Build history of the part. All positions in model axes, mm. A direction names the side the tool comes from. Coordinates: 2 decimals unless noted, no trailing zeros. Loops run counter-clockwise (first coordinate to the right, second up) from the corner with the lowest first, then second, coordinate; pieces in that order, holes last.
Item 1: Cut at A-A (y = 0). List the corners of the cut face in (x, z), and give its area (3 significant figures).
Item 2: Cut at C-C (x = 73.5). List the corners of the cut face in (y, z), and give its area (3 significant figures).
Item 3: Flat gauge pins, fed straight in: pin 1 (12 mm diameter, centred on y = -3.5, z = 58.5, fed in from +X); pin 2 (6.5 mm diameter, centred on x = 44.5, y = 28.5, fed in from -Z); pin 3 (5 mm diameter, centred on x = 4.5, z = 0, fed in from -Y). Where does each tip first touch, or does it go through?
Item 4: 3-axis set-ups, long thin cutter, end or side, ignore diameter. For faces 4 (the face through (5, -20, 1)), 5 (the face through (86, 11.6, 22.5)), 6 (the face through (49, 32.495, 0)): which of +Z, -Z, +X, -X, +Y, -Y reach the whole face in a straight line?
Item 5: Mould opens along Z. For faces 1 (the face through (17.75, -28.73, -69.28)), 2 (the face through (49, 28, 5)), 3 (the face through (10, 0, -45)) say: released by +Z, released by -Z, zero draft, split by the parting line, or undercut.
Item 6: Drill centre lines: line 1 along Y through (x, z) = (70, 0); line 2 along Y through (x, z) = (35.5, 0); line 3 along Z through (x, y) = (26, 0). Where is each one in solid material? Low to high.
Item 7: Cut at D-D (x = 23.5). List the corners of the cut face in (y, z), and give its area (3 significant figures).
Item 8: Cut at B-B (z = 0). List the corners of the cut face in (x, y), and give its area (3 significant figures).
from build123d import *

# Parameters (mm, degrees)
SKETCH1_R           = 75
BOSS_EXTRUDE1_DEPTH = 36
SKETCH2_R           = 50
BOSS_EXTRUDE2_DEPTH = 50
CUT_EXTRUDE2_DEPTH  = 10
CUT_EXTRUDE3_DEPTH  = 76
CHAMFER1_SIZE       = 1
CHAMFER2_SIZE       = 1


with BuildPart() as part:
    # Sketch1 → Boss-Extrude1 (new body)
    with BuildSketch(Plane(origin=(0, 0, 0), x_dir=(0, 0, -1), z_dir=(1, 0, 0))):
        Circle(SKETCH1_R)
    extrude(amount=BOSS_EXTRUDE1_DEPTH)

    # Sketch2 → Boss-Extrude2 (add)
    with BuildSketch(Plane(origin=(36, 0, 0), x_dir=(0, 0, -1), z_dir=(1, 0, 0))):
        Circle(SKETCH2_R)
    extrude(amount=BOSS_EXTRUDE2_DEPTH)

    # Sketch4 → Cut-Extrude2 (cut)
    with BuildSketch(Plane.ZY):
        with BuildLine():
            Line((-72.284161474, 20), (72.284161474, 20))
            ThreePointArc((72.284161474, 20), (75, 0), (72.284161474, -20))
            Line((72.284161474, -20), (-72.284161474, -20))
            ThreePointArc((-72.284161474, -20), (-75, 0), (-72.284161474, 20))
        make_face()
    extrude(amount=-CUT_EXTRUDE2_DEPTH, mode=Mode.SUBTRACT)

    # Sketch5 → Cut-Extrude3 (cut)
    with BuildSketch(Plane(origin=(86, 0, 0), x_dir=(0, 0, -1), z_dir=(1, 0, 0))):
        with BuildLine():
            Line((-5, 32.494897428), (5, 32.494897428))
            Line((5, 32.494897428), (5, 24.494897428))
            ThreePointArc((5, 24.494897428), (0, -25), (-5, 24.494897428))
            Line((-5, 24.494897428), (-5, 32.494897428))
        make_face()
    extrude(amount=-CUT_EXTRUDE3_DEPTH, mode=Mode.SUBTRACT)

    # Chamfer1
    chamfer1_edges = [part.edges().sort_by_distance(p)[0] for p in [
        (86, 0, 50),
    ]]
    chamfer(chamfer1_edges, length=CHAMFER1_SIZE)

    # Chamfer2
    chamfer2_edges = [part.edges().sort_by_distance(p)[0] for p in [
        (36, 0, 50),
    ]]
    chamfer(chamfer2_edges, length=CHAMFER2_SIZE)


solid = part.part
Filled sheet:
1. outline: (10, -75) - (36, -75) - (36, -51) - (37, -50) - (85, -50) - (86, -49) - (86, -25) - (10, -25) - close; (10, 25) - (86, 25) - (86, 49) - (85, 50) - (37, 50) - (36, 51) - (36, 75) - (10, 75) - close
1. area: 5,100 mm2
2. outline: circle Ø100 at (0, 0); hole (24.49, -5) - (32.49, -5) - (32.49, 5) - (24.49, 5) arc R25 ccw (long way) to start
2. area: 5,810 mm2
3. pin 1: stops at x = 36
3. pin 2: stops at z = -43.16
3. pin 3: stops at y = -75
4. face 4: +Z, -Z, -X
4. face 5: +Z, -Z, +X, +Y, -Y
4. face 6: +X
5. face 1: split by the parting line
5. face 2: undercut
5. face 3: zero draft
6. line 1: y = -50 to -25, 32.49 to 50
6. line 2: y = -75 to -25, 32.49 to 75
6. line 3: z = -75 to -25, 25 to 75
7. outline: circle Ø150 at (0, 0); hole (24.49, -5) - (32.49, -5) - (32.49, 5) - (24.49, 5) arc R25 ccw (long way) to start
7. area: 15,600 mm2
8. outline: (0, -75) - (36, -75) - (36, -51) - (37, -50) - (85, -50) - (86, -49) - (86, -25) - (10, -25) - (10, -20) - (0, -20) - close; (0, 20) - (10, 20) - (10, 32.49) - (86, 32.49) - (86, 49) - (85, 50) - (37, 50) - (36, 51) - (36, 75) - (0, 75) - close
8. area: 5,630 mm2
